Could you check a few things on this model? Use its own coordinates, in mm. A direction names the side the tool comes from. Coordinates: 2 decimals unless noted, no trailing zeros. Order: outer loops, then holes, each group sorted by start corner. A loop starts at its lowest first (then second) coordinate and runs counter-clockwise, first axis right, second up. Notation, with made-up numbers: (-13, -38) - (35, -38) arc R21 cw to (35, -31) - close; hole circle Ø9 at (47.25, 16.5). An arc over 180 degrees is marked (long way). One line per item, written item: value. Start each with the question number.
from build123d import *

# Parameters (mm, degrees)
F1_DEPTH = 600
F2_W     = 600
F2_H     = 280
F3_DEPTH = 400.001
F5_DEPTH = 700.001
F6_R     = 120
F7_DEPTH = 600.001
F8_W     = 220
F8_H     = 140
F9_DEPTH = 1200.001


with BuildPart() as f1:
    # F0 (on Front) → F1 (new body)
    with BuildSketch(Plane.XZ):
        Polygon((-70.953188, 0), (0, 0), (929.046812, 0), (929.046812, 500), (429.046812, 500), (429.046812, 200), (-270.953188, 200), (-270.953188, -200), (-70.953188, -200), align=None)
    extrude(amount=F1_DEPTH)

    # F2 (on face) → F3 (cut, through all)
    with BuildSketch(Plane.XY.offset(200)):
        with Locations((-270.953188, -300)):
            Rectangle(F2_W, F2_H)
    extrude(amount=-F3_DEPTH, mode=Mode.SUBTRACT)

    # F4 (on face) → F5 (cut, through all)
    with BuildSketch(Plane.XY.offset(500)):
        with BuildLine():
            ThreePointArc((529.046812, -450), (543.691473, -485.355339), (579.046812, -500))
            Line((579.046812, -500), (779.046812, -500))
            ThreePointArc((779.046812, -500), (814.402152, -485.355339), (829.046812, -450))
            Line((829.046812, -450), (829.046812, -150))
            ThreePointArc((829.046812, -150), (814.402152, -114.644661), (779.046812, -100))
            Line((779.046812, -100), (579.046812, -100))
            ThreePointArc((579.046812, -100), (543.691473, -114.644661), (529.046812, -150))
            Line((529.046812, -150), (529.046812, -450))
        make_face()
    extrude(amount=-F5_DEPTH, mode=Mode.SUBTRACT)

    # F6 (on face) → F7 (cut, through all)
    with BuildSketch(Plane.XZ.offset(600)):
        with Locations((679.046812, 250)):
            Circle(F6_R)
    extrude(amount=-F7_DEPTH, mode=Mode.SUBTRACT)

    # F8 (on face) → F9 (cut, through all)
    with BuildSketch(Plane.YZ.offset(929.046812)):
        with Locations((-300, 330)):
            Rectangle(F8_W, F8_H)
    extrude(amount=-F9_DEPTH, mode=Mode.SUBTRACT)


solid = f1.part
Q1. I want a section at D-D on y = -71.5. Please give me the cut outline in (x, z).
Q2. We'd pull the mould along X, two halves only. Please class faces 4 (the flat face through (29.047, -302, 101)), 5 (the flat face through (880, -190, 329)), 6 (the flat face through (680, -100, 430)): +X half, -X half, draft (parallel to the pull), parting line (faces both ways), or undercut.
Q3. If I drill on L1, parallel to X at y = -318, z = 15.5; L2, parallel to X at y = -57, z = 250; L3, parallel to Y at x = -146, z = 114, over which ranges is the centre line in solid material (lowest first)?
Q4. I want a section at B-B on z = 96. Please give me the cut outline in (x, y), then the cut area to 3 significant figures.
Q5. I want a section at A-A on y = -302. Please give me the cut outline in (x, z).
Q6. Which directions (+Z, -Z, +X, -X, +Y, -Y) give clear straight access to the entire face, cutting with the end or side of a thin tool? Please do faces 1 (the flat face through (480, -410, 329)), 2 (the flat face through (678, -500, 430)), 3 (the flat face through (422, -296, 0)).
Q7. I'm going to push a flat-ended pin straight in: pin 1 (1 mm diameter, centred on x = 150.5, y = -477.5, fed in from +Z). Where does the tip first touch, or does it pass through?
Q8. I want a section at C-C on z = -92.5. Please give me the cut outline in (x, y).
Values follow:
1. outline: (-270.95, -200) - (-70.95, -200) - (-70.95, 0) - (929.05, 0) - (929.05, 500) - (429.05, 500) - (429.05, 200) - (-270.95, 200) - close; hole circle Ø240 at (679.05, 250)
2. face 4: -X half
2. face 5: draft
2. face 6: undercut
3. L1: x = 29.05 to 529.05, 829.05 to 929.05
3. L2: x = 429.05 to 559.05, 799.05 to 929.05
3. L3: y = -600 to -440, -160 to 0
4. outline: (-270.95, -600) - (929.05, -600) - (929.05, 0) - (-270.95, 0) - (-270.95, -160) - (29.05, -160) - (29.05, -440) - (-270.95, -440) - close; hole (529.05, -450) arc R50 ccw to (579.05, -500) - (779.05, -500) arc R50 ccw to (829.05, -450) - (829.05, -150) arc R50 ccw to (779.05, -100) - (579.05, -100) arc R50 ccw to (529.05, -150) - close
4. area: 518,000 mm^2
5. outline: (29.05, 0) - (529.05, 0) - (529.05, 260) - (429.05, 260) - (429.05, 200) - (29.05, 200) - close; (429.05, 400) - (529.05, 400) - (529.05, 500) - (429.05, 500) - close; (829.05, 0) - (929.05, 0) - (929.05, 260) - (829.05, 260) - close; (829.05, 400) - (929.05, 400) - (929.05, 500) - (829.05, 500) - close
6. face 1: +X, -X
6. face 2: +Z, -Z
6. face 3: -Z, +X, +Y, -Y
7. pin 1: stops at z = 200
8. outline: (-270.95, -600) - (-70.95, -600) - (-70.95, -440) - (-270.95, -440) - close; (-270.95, -160) - (-70.95, -160) - (-70.95, 0) - (-270.95, 0) - close
